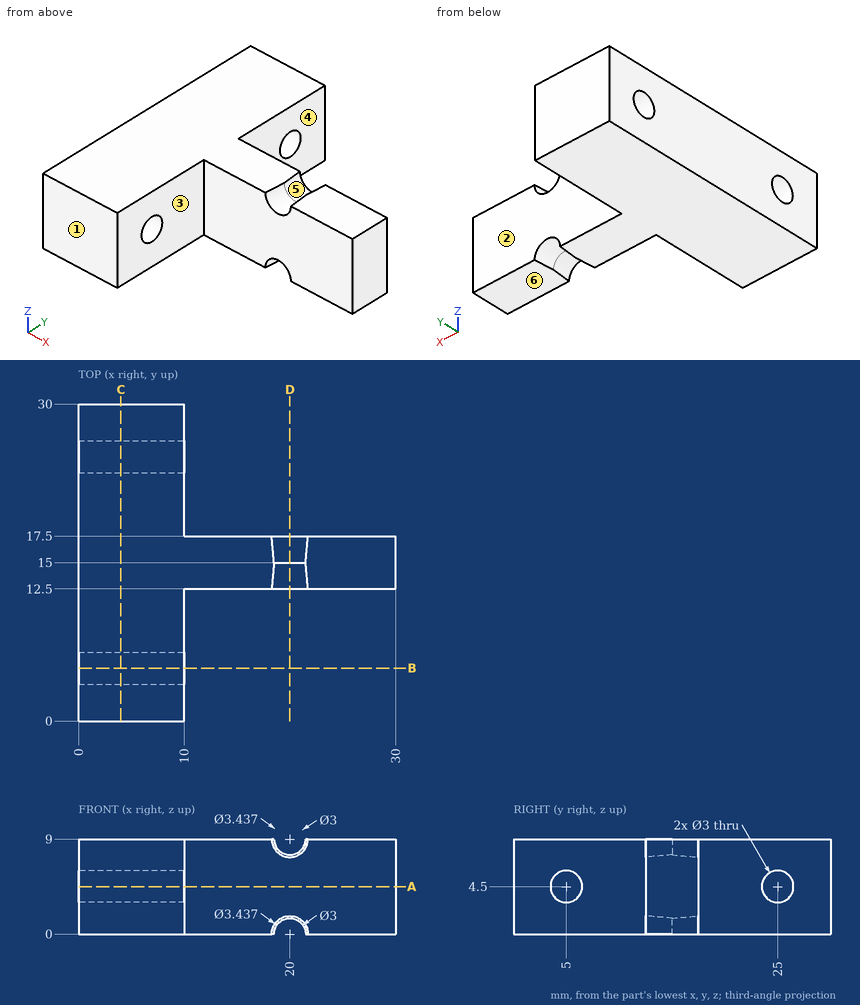
Drawing for the job (mm, zero at the part's lowest x, y, z). A direction names the side the tool comes from. Round coordinates to 2 decimals unless told otherwise and drop trailing zeros. Write each loop counter-clockwise with the first axis right and the second up, starting at its lowest first coordinate (ties: lowest second). Pieces come first, ordered by that corner, then holes.
Item 1: Band-saw the part on D-D on x = 20. Write the cut outline in (y, z), then the cut area to 3 significant figures.
Filled in:
outline: (12.5, 1.72) - (15, 1.5) - (17.5, 1.72) - (17.5, 7.28) - (15, 7.5) - (12.5, 7.28) - close
area: 28.9 mm2
Item 2: Mould opens along X. For the marked faces 4, 5 and 6 say: released by +X, released by -X, zero draft, split by the parting line, or undercut.
Filled in:
face 4: released by +X
face 5: undercut
face 6: zero draft
Item 3: Band-saw the part on B-B on y = 5. Write the cut outline in (x, z), then the cut area to 3 significant figures.
Filled in:
outline: (0, 0) - (10, 0) - (10, 3) - (0, 3) - close; (0, 6) - (10, 6) - (10, 9) - (0, 9) - close
area: 60.0 mm2
Item 4: Band-saw the part on A-A on z = 4.5. Write the cut outline in (x, y).
Filled in:
outline: (0, 0) - (10, 0) - (10, 3.5) - (0, 3.5) - close; (0, 6.5) - (10, 6.5) - (10, 12.5) - (30, 12.5) - (30, 17.5) - (10, 17.5) - (10, 23.5) - (0, 23.5) - close; (0, 26.5) - (10, 26.5) - (10, 30) - (0, 30) - close
Item 5: Band-saw the part on C-C on x = 4. Write the cut outline in (y, z).
Filled in:
outline: (0, 0) - (30, 0) - (30, 9) - (0, 9) - close; hole circle Ø3 at (5, 4.5); hole circle Ø3 at (25, 4.5)
Item 6: Drill centre lines: L1, parallel to Y at x = 7, z = 4.5; L2, parallel to Z at x = 6.5, y = 5; L3, parallel to X at y = 11.75, z = 3.5. Where is each one in solid material? Low to high.
Filled in:
L1: y = 0 to 3.5, 6.5 to 23.5, 26.5 to 30
L2: z = 0 to 3, 6 to 9
L3: x = 0 to 10
Item 7: Drop flat-ended pins along their axis: pin 1 Ø2.5 at (y, z) = (26, 2.5) entering from +X; pin 2 Ø1 at (x, z) = (14.5, 7.5) entering from +Y; pin 3 Ø2 at (x, z) = (15, 2.5) entering from -Y. Give the stop position or say it passes through.
Filled in:
pin 1: stops at x = 10
pin 2: stops at y = 17.5
pin 3: stops at y = 12.5
Item 8: Tool access for the marked faces 1, 2 and 3: list every direction of +Z, -Z, +X, -X, +Y, -Y with a clear straight run to the whole face (end or side of a thin tool).
Filled in:
face 1: +Z, -Z, +X, -X, -Y
face 2: +Z, -Z, +X, +Y
face 3: +Z, -Z, +X, -Y
